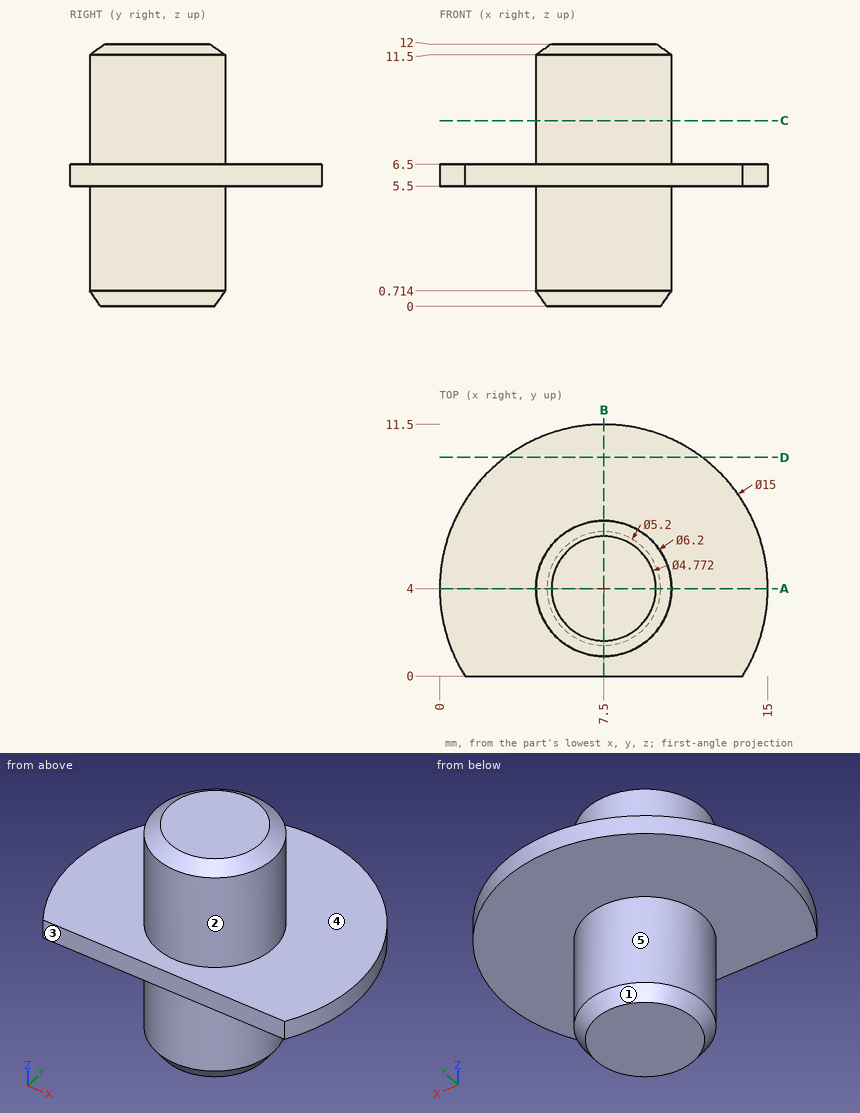
For this review, use the dimensioned drawing (mm, ordinates from the lowest corner) and the shaded views. A direction names the side the tool comes from. Coordinates: 2 decimals unless noted, no trailing zeros. Loops run counter-clockwise (first coordinate to the right, second up) from the corner with the lowest first, then second, coordinate; pieces in that order, holes last. Notation, with made-up numbers: (13, 18) -> (23, 18) arc R34 ccw to (23, 54) -> close; hole circle Ø11 at (64, -35). An arc over 180 degrees is marked (long way). Use a Markdown table: item, result. Add a question column.
Item 1: The part is to be moulded in two halves that separate along Y. For the marked faces 3, 4 and 5, say which applies: +Y half, -Y half, draft (parallel to the pull), parting line (faces both ways), or undercut.
Item 2: Wall thickness on L1, parallel to Z at x = 12.5, y = 9.25; L2, parallel to Y at x = 9, z = 3.5; L3, parallel to Z at x = 10.5, y = 4: over which ranges is each line inside the solid? List them lowest first. Write a range as from..to.
Item 3: We need section B-B, the plane x = 7.5. Write out the cut boundary in (y, z).
Item 4: We need section D-D, the plane y = 10. Write out the cut boundary in (x, z).
Item 5: Machinability: for the marked faces 1 and 2, which of the approach directions +Z, -Z, +X, -X, +Y, -Y give a long, thin tool a straight path to every point of the face, cutting with its end or side? Answer none if there is none.
Item 6: We need section A-A, the plane y = 4. Write out the cut boundary in (x, z).
Item 7: Clearance check with flat-ended pins moving along their axes: P1, Ø3, axis at x = 12, z = 4.5, coming from the -Y side; P2, Ø6, axis at y = 8.5, z = 5, coming from the +X side; P3, Ø2, axis at x = 5, y = 7.5, coming from the -Z side. State where each tip first meets the part, or that it passes through.
Item 8: We need section C-C, the plane z = 8.5. Write out the cut boundary in (x, y).
Numbers:
| question | item | result |
|---|---|---|
| 1 | face 3 | -Y half |
| 1 | face 4 | draft |
| 1 | face 5 | parting line |
| 2 | L1 | z = 5.5..6.5 |
| 2 | L2 | y = 1.29..6.71 |
| 2 | L3 | z = 0.57..11.57 |
| 3 | outline | (0, 5.5) -> (0.9, 5.5) -> (0.9, 0.71) -> (1.4, 0) -> (6.6, 0) -> (7.1, 0.71) -> (7.1, 5.5) -> (11.5, 5.5) -> (11.5, 6.5) -> (7.1, 6.5) -> (7.1, 11.5) -> (6.39, 12) -> (1.61, 12) -> (0.9, 11.5) -> (0.9, 6.5) -> (0, 6.5) -> close |
| 4 | outline | (3, 5.5) -> (12, 5.5) -> (12, 6.5) -> (3, 6.5) -> close |
| 5 | face 1 | -Z |
| 5 | face 2 | +Z |
| 6 | outline | (0, 5.5) -> (4.4, 5.5) -> (4.4, 0.71) -> (4.9, 0) -> (10.1, 0) -> (10.6, 0.71) -> (10.6, 5.5) -> (15, 5.5) -> (15, 6.5) -> (10.6, 6.5) -> (10.6, 11.5) -> (9.89, 12) -> (5.11, 12) -> (4.4, 11.5) -> (4.4, 6.5) -> (0, 6.5) -> close |
| 7 | P1 | stops at y = 0 |
| 7 | P2 | stops at x = 14.84 |
| 7 | P3 | stops at z = 5.5 |
| 8 | outline | circle Ø6.2 at (7.5, 4) |
